Can you work these out from the drawing? Everything is in mm from the part's minimum corner. A direction names the side the tool comes from. Round coordinates to 2 decimals unless told otherwise and drop trailing zeros. Loops run counter-clockwise (first coordinate to the right, second up) from the corner with the lowest first, then second, coordinate; pieces in that order, holes last. Notation, with made-up numbers: (57, 44) -> (114, 44) arc R8 ccw to (114, 56) -> close; hole circle Ø7 at (-4, 35). An arc over 180 degrees is marked (long way). One line per item, written item: value.
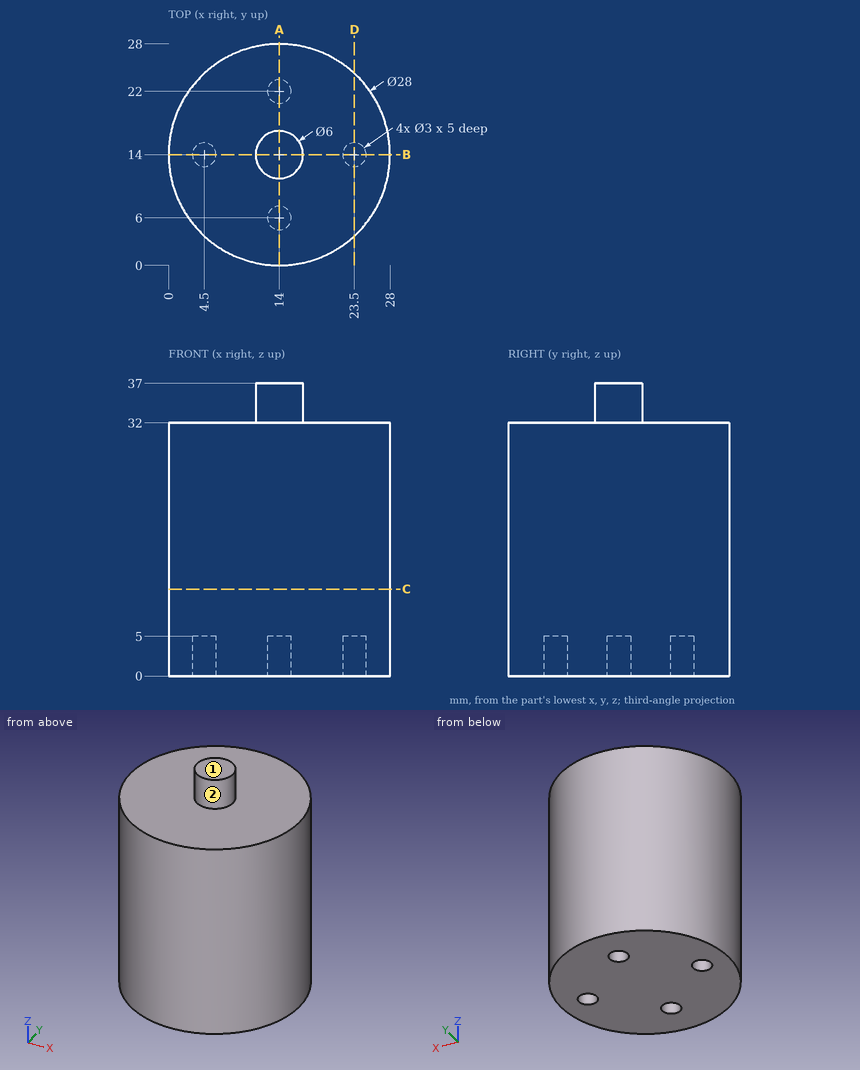
(1) Imagine slicing it at C-C on z = 11. Write out the boundary of the cut face in (x, y), then the cut area to 3 significant figures.
Results below:
outline: circle Ø28 at (14, 14)
area: 616 mm²
(2) Imagine slicing it at A-A on x = 14. Write out the boundary of the cut face in (y, z).
Results below:
outline: (0, 0) -> (4.5, 0) -> (4.5, 5) -> (7.5, 5) -> (7.5, 0) -> (20.5, 0) -> (20.5, 5) -> (23.5, 5) -> (23.5, 0) -> (28, 0) -> (28, 32) -> (17, 32) -> (17, 37) -> (11, 37) -> (11, 32) -> (0, 32) -> close
(3) Imagine slicing it at B-B on y = 14. Write out the boundary of the cut face in (x, z), then the cut area to 3 significant figures.
Results below:
outline: (0, 0) -> (3, 0) -> (3, 5) -> (6, 5) -> (6, 0) -> (22, 0) -> (22, 5) -> (25, 5) -> (25, 0) -> (28, 0) -> (28, 32) -> (17, 32) -> (17, 37) -> (11, 37) -> (11, 32) -> (0, 32) -> close
area: 896 mm²
(4) For pin 1 Ø3.5 at (x, y) = (14, 6) entering from +Z; pin 2 Ø5 at (y, z) = (8, 24) entering from +X; pin 3 Ø1.8 at (x, y) = (4.5, 14) entering from -Z, each with a flat end and sliding along its axis, tell me the tip position at first contact or that it passes through.
Results below:
pin 1: stops at z = 32
pin 2: stops at x = 27.56
pin 3: stops at z = 5
(5) Imagine slicing it at D-D on x = 23.5. Write out the boundary of the cut face in (y, z).
Results below:
outline: (3.72, 0) -> (12.5, 0) -> (12.5, 5) -> (15.5, 5) -> (15.5, 0) -> (24.28, 0) -> (24.28, 32) -> (3.72, 32) -> close
(6) On a 3-axis mill with a long thin cutter (end or side, diameter ignored), from which of +Z, -Z, +X, -X, +Y, -Y can I reach the whole of each face in a straight line? I mean the marked faces 1 and 2. Say none if no direction works.
Results below:
face 1: +Z, +X, -X, +Y, -Y
face 2: +Z
(7) Please list where these lines run through material, in increasing order: L1, parallel to Y at x = 14, z = 1.2; L2, parallel to Y at x = 14.5, z = 23.5; L3, parallel to Z at x = 7.5, y = 22.
Results below:
L1: y = 0 to 4.5, 7.5 to 20.5, 23.5 to 28
L2: y = 0.01 to 27.99
L3: z = 0 to 32
